Can you work these out from the drawing? Everything is in mm from the part's minimum corner. A direction names the side the tool comes from. Give positions to 0.01 mm unless a question says otherwise; leave off trailing zeros. Order: outer loops, then holes, each group sorted by start corner. A loop starts at its lowest first (then second) coordinate and runs counter-clockwise, first axis right, second up. Notation, with made-up numbers: M 57,-14.5 L 116,-14.5 A23 cw 116,-1.5 Z; hole C 50.25,73 d5. An arc over 180 degrees is marked long. Answer as a JSON object with one key per item and string values.
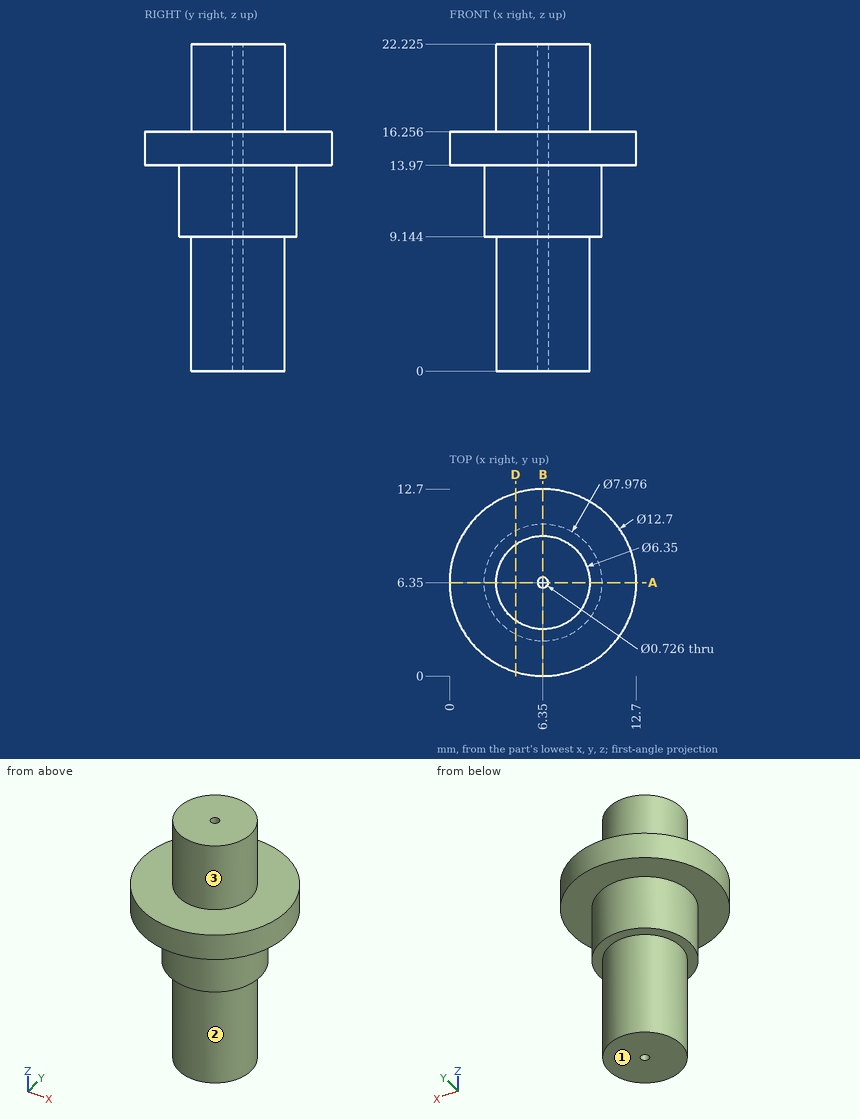
1) For the marked faces 1, 2 and 3, which set-ups out of +Z, -Z, +X, -X, +Y, -Y let a thin tool reach every point of the face, with its end or its side?
Results found:
{"face 1": "-Z, +X, -X, +Y, -Y", "face 2": "-Z", "face 3": "+Z"}
2) I want a section at D-D on x = 4.5. Write out the boundary of the cut face in (y, z) (1 decimal).
Results found:
{"outline": "M 0.3,14 L 2.8,14 L 2.8,9.1 L 3.8,9.1 L 3.8,0 L 8.9,0 L 8.9,9.1 L 9.9,9.1 L 9.9,14 L 12.4,14 L 12.4,16.3 L 8.9,16.3 L 8.9,22.2 L 3.8,22.2 L 3.8,16.3 L 0.3,16.3 Z"}
3) I want a section at A-A on y = 6.35. Write out the boundary of the cut face in (x, z) (1 decimal).
Results found:
{"outline": "M 0,14 L 2.4,14 L 2.4,9.1 L 3.2,9.1 L 3.2,0 L 6,0 L 6,22.2 L 3.2,22.2 L 3.2,16.3 L 0,16.3 Z; M 6.7,0 L 9.5,0 L 9.5,9.1 L 10.3,9.1 L 10.3,14 L 12.7,14 L 12.7,16.3 L 9.5,16.3 L 9.5,22.2 L 6.7,22.2 Z"}
4) I'm going to push flat-ended pins straight in: pin 1 Ø2 at (x, y) = (7, 3) entering from +Z (3 decimals); pin 2 Ø5 at (y, z) = (9, 9) entering from +X (1 decimal); pin 3 Ø1 at (x, y) = (9, 2) entering from +Z; pin 4 Ø1.5 at (x, z) = (3.5, 14) entering from -Y. Where does each tip first touch, or does it pass through?
Results found:
{"pin 1": "stops at z = 22.225", "pin 2": "stops at x = 10.3", "pin 3": "stops at z = 16.26", "pin 4": "stops at y = 0.36"}
5) I need wall thicknesses on L1, parallel to Y at x = 6.35, z = 12.75; L2, parallel to Y at x = 6.35, z = 15; L3, parallel to Z at x = 8.25, y = 3.25. Which ranges of each line are inside material? Lowest first, please.
Results found:
{"L1": "y = 2.36 to 5.99, 6.71 to 10.34", "L2": "y = 0 to 5.99, 6.71 to 12.7", "L3": "z = 9.14 to 16.26"}
